Input: part model. Units: mm. Frame: model coordinates. A direction names the side the tool comes from. Round coordinates to 2 decimals unless told otherwise and drop trailing zeros. Loops run counter-clockwise (first coordinate to the right, second up) from the corner with the lowest first, then second, coordinate; pieces in that order, holes last.
(1) Access query for faces 1 (the face through (-2.17, -9.76, 9.68)), 2 (the face through (-3, 0, 0)), 3 (the face through (7, -10, 19.5)). Directions: +Z, -Z, +X, -X, +Y, -Y. A direction counts if a zero-diameter tool reaches every point of the face in a straight line with its end or side. Return the directions, or none.
(2) Line query: line 1 (Z direction, x = -8.5, y = 4); line 2 (Y direction, x = 8.25, z = 3.5); line 3 (Y direction, x = -4.5, z = 9.75). Output: solid intervals per line, ascending.
(3) Cut plane B-B, the plane z = 17.75. Output: boundary loops of the cut face in (x, y), and give its area (3 significant figures).
(4) Draft query along Z for faces 4 (the face through (8.73, 6.69, 9.88)), 5 (the face through (-0.933, 0.832, 1.514)), 6 (the face through (4, -2, 5)). Return one class per face: released by +Z, released by -Z, zero draft, split by the parting line, or undercut.
(5) First-contact query: pin 1 Ø2 at (x, y) = (9.5, 2.5) entering from +Z; pin 2 Ø6.5 at (x, y) = (1.92, 5.9) entering from +Z; pin 3 Ø10 at (x, y) = (-1, -5) entering from +Z. Flat tips, straight axial feed; report the tip coordinate or a pass-through.
(6) Cut plane A-A, the plane z = 7.25. Output: boundary loops of the cut face in (x, y).
from build123d import *

# Parameters (mm, degrees)
ESBO_O1_R                = 12.5
RESSALTO_EXTRUS_O1_DEPTH = 21
ESBO_O4_W                = 18
ESBO_O4_H                = 1.4999999999999982
ESBO_O5_R                = 9.25
CORTE_EXTRUS_O1_DEPTH    = 14
CORTE_EXTRUS_O2_DEPTH    = 17
ESBO_O7_R                = 2.499999999999999
ESBO_O7_R_2              = 2.5000000000000018
ESBO_O7_R_3              = 2.5
ESBO_O7_R_4              = 2.500000000000001
ESBO_O7_R_5              = 2.5000000000000004
CORTE_EXTRUS_O3_DEPTH    = 17
ESBO_O11_R               = 10
CORTE_EXTRUS_O4_DEPTH    = 23.54994456755936
CHANFRO3_SIZE            = 0.5
FILETE2_R                = 1
ESBO_O12_R               = 4.25
CORTE_EXTRUS_O5_DEPTH    = 4.5
CORTE_EXTRUS_O6_START    = -2
ESBO_O13_R               = 9.999999999998892
CORTE_EXTRUS_O6_DEPTH    = 2
ESBO_O14_R               = 10.5
CORTE_EXTRUS_O7_DEPTH    = 6
CHANFRO5_SIZE            = 0.5
FILETE3_R                = 1.5
FILETE4_R                = 0.5


# Some blends are built 0.0001 mm under size
with BuildPart() as part:
    # Esboço1 → Ressalto-extrusão1 (new body)
    with BuildSketch(Plane.XY):
        with Locations(Location((0, 0, 0), (0, 0, 180))):
            Circle(ESBO_O1_R)
    extrude(amount=RESSALTO_EXTRUS_O1_DEPTH)

    # Esboço4 → Corte-Revolução1 (revolve, cut)
    with BuildSketch(Plane(origin=(0, 0, 0), x_dir=(0, 0, -1), z_dir=(1, 0, 0)), mode=Mode.PRIVATE) as corte_revolu_o1_sk:
        with Locations((-10.5, -11.750000000000004)):
            Rectangle(ESBO_O4_W, ESBO_O4_H)
    revolve(corte_revolu_o1_sk.sketch.rotate(Axis((0, 0, -2.777032731116021), (0, 0, 1)), 270), axis=Axis((0, 0, -2.777032731116021), (0, 0, 1)), mode=Mode.SUBTRACT)

    # Esboço5 → Corte-extrusão1 (cut)
    with BuildSketch(Plane.XY.offset(21)):
        Circle(ESBO_O5_R)
    extrude(amount=-CORTE_EXTRUS_O1_DEPTH, mode=Mode.SUBTRACT)

    # Esboço6 → Corte-extrusão2 (cut)
    with BuildSketch(Plane.XY.offset(7.000000000000001)):
        with BuildLine():
            Line((-1.6492922297361152, 0.04832329595623431), (-0.1960424852505637, 1.6383123462810085))
            ThreePointArc((-0.1960424852505637, 1.6383123462810085), (1.2179209118912084, -1.1131795238765794), (-1.6492922297361152, 0.04832329595623431))
        make_face()
    extrude(amount=-CORTE_EXTRUS_O2_DEPTH, mode=Mode.SUBTRACT)

    # Esboço7 → Corte-extrusão3 (cut)
    with BuildSketch(Plane.XY.offset(7.000000000000001)):
        with Locations((6.2, 0)):
            Circle(ESBO_O7_R)
        with Locations((1.9159053651246736, -5.896550401029952)):
            Circle(ESBO_O7_R_2)
        with Locations((-5.015905365124674, -3.644268564213333)):
            Circle(ESBO_O7_R_3)
        with Locations((-5.0159053651246746, 3.644268564213335)):
            Circle(ESBO_O7_R_4)
        with Locations((1.9159053651246742, 5.8965504010299545)):
            Circle(ESBO_O7_R_5)
    extrude(amount=-CORTE_EXTRUS_O3_DEPTH, mode=Mode.SUBTRACT)

    # Esboço11 → Corte-extrusão4 (cut, through all)
    with BuildSketch(Plane.XY.offset(7.000000000000001)):
        Circle(ESBO_O11_R)
    extrude(amount=CORTE_EXTRUS_O4_DEPTH, mode=Mode.SUBTRACT)

    # Chanfro3
    chanfro3_edges = [part.edges().sort_by_distance(p)[0] for p in [
        (-0.9226673574933396, 0.8433178211186214, 0),
        (1.2179209118912089, -1.1131795238765791, 0),
    ]]
    chamfer(chanfro3_edges, length=CHANFRO3_SIZE)

    # Filete2
    filete2_edges = [part.edges().sort_by_distance(p)[0] for p in [
        (11.000000000000004, -3.79e-15, 19.5),
    ]]
    fillet(filete2_edges, radius=FILETE2_R)

    # Esboço12 → Corte-extrusão5 (cut)
    with BuildSketch(Plane.XY.offset(7.000000000000001)):
        Circle(ESBO_O12_R)
    extrude(amount=-CORTE_EXTRUS_O5_DEPTH, mode=Mode.SUBTRACT)

    # Esboço13 → Corte-extrusão6 (cut)
    with BuildSketch(Plane.XY.offset(7.000000000000001).offset(CORTE_EXTRUS_O6_START)):
        Circle(ESBO_O13_R)
    extrude(amount=CORTE_EXTRUS_O6_DEPTH, mode=Mode.SUBTRACT)

    # Esboço14 → Corte-extrusão7 (cut)
    with BuildSketch(Plane.XY.offset(21)):
        Circle(ESBO_O14_R)
    extrude(amount=-CORTE_EXTRUS_O7_DEPTH, mode=Mode.SUBTRACT)

    # Chanfro5
    chanfro5_edges = [part.edges().sort_by_distance(p)[0] for p in [
        (-10, -3.6e-16, 15),
    ]]
    chamfer(chanfro5_edges, length=CHANFRO5_SIZE - 0.0001)  # a hair under: the kernel refuses the full size

    # Filete3
    filete3_edges = [part.edges().sort_by_distance(p)[0] for p in [
        (-10.49999999999999, -2.18e-15, 21),
    ]]
    fillet(filete3_edges, radius=FILETE3_R)

    # Filete4
    # the kernel refuses this fillet: 0.5 mm, written as the material it takes off along each edge
    with BuildSketch(Plane(origin=(0.0348414521611502, 4.24985718268406, 2.500000000000001), x_dir=(-0.5385482675790525, 0.8425946614402451, 0), z_dir=(0, 0, 1))) as filete4_piece_1:
        with BuildLine():
            CenterArc((0.823792647207476, 0.4943596381730637), FILETE4_R, 157.42158231985286, 103.96421233199169)
            ThreePointArc((0.3621151927317683, 0.6863334072896572), (0.19675498821110124, 0.3348846296367101), (0, 0))
            ThreePointArc((0, 0), (0.3744512032761266, 0.02820180913468155), (0.7489024065522512, 3e-17))
        make_face()
    extrude(amount=4.440007987691346, mode=Mode.SUBTRACT)
    with BuildSketch(Plane(origin=(-4.031087766088941, 1.346414283230858, 2.500000000000001), x_dir=(-0.9677757103313676, -0.2518137694658835, 0), z_dir=(0, 0, 1))) as filete4_piece_2:
        with BuildLine():
            CenterArc((0.8237926472074756, 0.4943596381730638), FILETE4_R, 157.42158231985286, 103.96421233199163)
            ThreePointArc((0.36211519273176773, 0.6863334072896573), (0.19675498821110218, 0.3348846296367097), (0, 0))
            ThreePointArc((0, 0), (0.3744512032761257, 0.02820180913468181), (0.7489024065522503, 3e-17))
        make_face()
    extrude(amount=4.440007987691345, mode=Mode.SUBTRACT)
    with BuildSketch(Plane(origin=(-2.5261907032380004, -3.417727392709064, 2.500000000000001), x_dir=(-0.059570014892305595, -0.9982241298053911, 0), z_dir=(0, 0, 1))) as filete4_piece_3:
        with BuildLine():
            CenterArc((0.8237926472074754, 0.4943596381730636), FILETE4_R, 157.42158231985266, 103.9642123319918)
            ThreePointArc((0.3621151927317685, 0.6863334072896586), (0.19675498821109988, 0.33488462963670823), (0, 0))
            ThreePointArc((0, 0), (0.37445120327612497, 0.02820180913468126), (0.7489024065522498, 0))
        make_face()
    extrude(amount=4.44000798769135, mode=Mode.SUBTRACT)
    with BuildSketch(Plane(origin=(4.052620967741936, 1.2801419030007621, 2.500000000000001), x_dir=(0.6349345763851404, 0.7725659089751646, 0), z_dir=(0, 0, 1))) as filete4_piece_4:
        with BuildLine():
            CenterArc((0.8237926472074759, 0.4943596381730635), FILETE4_R, 157.42158231985277, 103.96421233199169)
            ThreePointArc((0.36211519273176856, 0.6863334072896574), (0.19675498821110185, 0.33488462963671034), (0, 0))
            ThreePointArc((0, 0), (0.37445120327612536, 0.0282018091346815), (0.7489024065522507, 1e-17))
        make_face()
    extrude(amount=4.440007987691347, mode=Mode.SUBTRACT)
    with BuildSketch(Plane(origin=(2.4698160494238595, -3.458685976206616, 2.500000000000001), x_dir=(0.9309594164175853, -0.36512267114413594, 0), z_dir=(0, 0, 1))) as filete4_piece_5:
        with BuildLine():
            CenterArc((0.8237926472074742, 0.49435963817306355), FILETE4_R, 157.4215823198528, 103.96421233199175)
            ThreePointArc((0.36211519273176695, 0.6863334072896573), (0.19675498821110182, 0.3348846296367097), (0, 0))
            ThreePointArc((0, 0), (0.374451203276125, 0.0282018091346814), (0.7489024065522494, 4e-17))
        make_face()
    extrude(amount=4.440007987691345, mode=Mode.SUBTRACT)
    with BuildSketch(Plane(origin=(2.469816049423857, 3.4586859762066187, 2.500000000000001), x_dir=(0.7573556902798542, -0.6530025715115719, 0), z_dir=(0, 0, 1))) as filete4_piece_6:
        with BuildLine():
            CenterArc((0.8216504418457475, 0.4979119689888876), FILETE4_R, 160.79770494401825, 103.96421233199163)
            ThreePointArc((0.34946884369362086, 0.662364206330018), (0.1996774167699546, 0.3180219723627336), (0, 0))
            ThreePointArc((0, 0), (0.38800159753826985, 0.01774826359445502), (0.776003195076539, -3e-17))
        make_face()
    extrude(amount=4.440007987691348, mode=Mode.SUBTRACT)
    with BuildSketch(Plane(origin=(4.052620967741936, -1.2801419030007621, 2.500000000000001), x_dir=(-0.3870065717105284, -0.9220769563614871, 0), z_dir=(0, 0, 1))) as filete4_piece_7:
        with BuildLine():
            CenterArc((0.8216504418457483, 0.4979119689888879), FILETE4_R, 160.7977049440181, 103.96421233199175)
            ThreePointArc((0.3494688436936216, 0.6623642063300196), (0.19967741676995576, 0.3180219723627358), (0, 0))
            ThreePointArc((0, 0), (0.38800159753827046, 0.01774826359445508), (0.7760031950765397, 0))
        make_face()
    extrude(amount=4.440007987691349, mode=Mode.SUBTRACT)
    with BuildSketch(Plane(origin=(0.0348414521611462, -4.24985718268406, 2.500000000000001), x_dir=(-0.9965389054665341, 0.08312767223712024, 0), z_dir=(0, 0, 1))) as filete4_piece_8:
        with BuildLine():
            CenterArc((0.8216504418457475, 0.4979119689888879), FILETE4_R, 160.79770494401836, 103.96421233199152)
            ThreePointArc((0.3494688436936206, 0.6623642063300171), (0.19967741676995457, 0.31802197236273494), (0, 0))
            ThreePointArc((0, 0), (0.3880015975382697, 0.01774826359445501), (0.776003195076539, -1e-17))
        make_face()
    extrude(amount=4.440007987691348, mode=Mode.SUBTRACT)
    with BuildSketch(Plane(origin=(-4.031087766088943, -1.3464142832308554, 2.500000000000001), x_dir=(-0.9677757103313678, 0.2518137694658824, 0), z_dir=(0, 0, 1))) as filete4_piece_9:
        with BuildLine():
            CenterArc((0.8237926472074728, -0.49435963817306383), FILETE4_R, 98.61420534815544, 103.9642123319918)
            ThreePointArc((0.36211519273176607, -0.686333407289658), (0.19675498821110143, -0.334884629636712), (0, 0))
            ThreePointArc((0, 0), (0.37445120327612447, -0.02820180913468116), (0.7489024065522482, -3e-17))
        make_face()
    extrude(amount=4.440007987691345, mode=Mode.SUBTRACT)
    with BuildSketch(Plane(origin=(-2.5261907032380004, 3.4177273927090632, 2.500000000000001), x_dir=(0.8550781298766168, 0.5184991724262514, 0), z_dir=(0, 0, 1))) as filete4_piece_10:
        with BuildLine():
            CenterArc((0.8216504418457481, 0.49791196898888734), FILETE4_R, 160.79770494401822, 103.96421233199158)
            ThreePointArc((0.3494688436936213, 0.6623642063300179), (0.19967741676995546, 0.31802197236273533), (0, 0))
            ThreePointArc((0, 0), (0.3880015975382698, 0.01774826359445526), (0.7760031950765391, -4e-17))
        make_face()
    extrude(amount=4.440007987691348, mode=Mode.SUBTRACT)


solid = part.part
Reported:
1. face 1: +Z
1. face 2: -Z, +X, -X, +Y, -Y
1. face 3: none
2. line 1: z = 0 to 5
2. line 2: y = -7.28 to -1.43, 1.43 to 7.28
2. line 3: y = -10.04 to -8.93, 8.93 to 10.04
3. outline: circle Ø22 at (0, 0); hole circle Ø21 at (0, 0)
3. area: 33.8 mm2
4. face 4: undercut
4. face 5: zero draft
4. face 6: released by +Z
5. pin 1: stops at z = 20.43
5. pin 2: stops at z = 5
5. pin 3: stops at z = 14.6
6. outline: circle Ø22 at (0, 0); hole circle Ø20 at (0, 0)
